from build123d import *

# Parameters (mm, degrees)
SKETCH1_R           = 1.75
BOSS_EXTRUDE1_DEPTH = 5


with BuildPart() as part:
    # Sketch1 → Boss-Extrude1 (new body)
    with BuildSketch(Plane.XY):
        with BuildLine():
            Line((-93.75, -249.14706128), (-98.75, -249.14706128))
            Line((-98.75, -249.14706128), (-98.75, -275.963602955))
            Line((-98.75, -275.963602955), (-93.75, -275.963602955))
            add(Edge.make_bspline(
                [(-93.75, -275.963602955), (-85.328784133, -309.023467032), (-87.242655609, -343.164760507), (-85.696102167, -376.929671114)],
                knots=[0, 0, 0, 0, 1, 1, 1, 1], degree=3))
            Line((-85.696102167, -376.929671114), (82.9, -376.929671114))
            add(Edge.make_bspline(
                [(82.9, -274.035506052), (82.9, -308.333561073), (82.9, -342.631616093), (82.9, -376.929671114)],
                knots=[0, 0, 0, 0, 1, 1, 1, 1], degree=3))
            Line((82.9, -274.035506052), (82.9, -262.713680137))
            ThreePointArc((82.9, -262.713680137), (82.607106781, -262.006573355), (81.9, -261.713680137))
            Line((81.9, -261.713680137), (77.9, -261.713680137))
            add(Edge.make_bspline(
                [(77.9, -261.713680137), (75.588198468, -253.598889885), (76.340151595, -245.239667724), (76.055808767, -236.957982208)],
                knots=[0, 0, 0, 0, 1, 1, 1, 1], degree=3))
            Line((76.055808767, -236.957982208), (-91.666234566, -236.957982208))
            add(Edge.make_bspline(
                [(-93.75, -249.14706128), (-91.542697993, -245.516719889), (-91.581655695, -241.056968833), (-91.666234566, -236.957982208)],
                knots=[0, 0, 0, 0, 1, 1, 1, 1], degree=3))
        make_face()
        with Locations((-96.249351551, -269.713963286)):
            Circle(SKETCH1_R, mode=Mode.SUBTRACT)
        with Locations((-96.243654126, -254.713964368)):
            Circle(SKETCH1_R, mode=Mode.SUBTRACT)
        with Locations((80.4, -267.874593094)):
            Circle(SKETCH1_R, mode=Mode.SUBTRACT)
    extrude(amount=BOSS_EXTRUDE1_DEPTH)


solid = part.part
Geometry: final body of the model. Coordinates: model frame, mm. A direction names the side the tool comes from. Coordinates: 2 decimals unless noted, no trailing zeros. One line per item, written item: value. Start each with the question number.
1) Pin query (flat end, axial travel): P1, Ø2, axis at x = -96.24, y = -254.71, coming from the +Z side; P2, Ø2, axis at y = -310.5, z = 1, coming from the -X side; P3, Ø1.5, axis at y = -362.5, z = 4.5, coming from the -X side; P4, Ø1.5, axis at x = -97.5, z = 1.5, coming from the -Y side. Return the tip coordinate at first contact, or that it passes through.
2) Material intervals for L1, parallel to Y at x = 80.4, z = 1.3; L2, parallel to X at y = -303, z = 3.6; L3, parallel to X at y = -249, z = 1.4, sorted ascending. Write a range as from..to.
3) Reachability of faces 1 (the flat face through (-96, -275.964, 2)), 2 (the flat face through (80, -261.714, 2)), 3 (the flat face through (-9, -306, 0)) from +Z, -Z, +X, -X, +Y, -Y: full face, straight path, thin tool, end or side. Return the list, or none.
4) Cut plane A-A (z = 3.6). Count the separate pieces of the cut face and the enclosed holes in it, then the cut area to 3 significant figures.
5) Draft query along Y for faces 4 (the cylindrical face through (79.01, -268.94, 2.46)), 5 (the flat face through (-98.75, -262, 2)), 6 (the flat face through (-96, -249.147, 2)). Return one class per face: released by +Y, released by -Y, zero draft, split by the parting line, or undercut.
Evaluation:
1. P1: through
1. P2: x = -88.25
1. P3: x = -86.2
1. P4: y = -275.96
2. L1: -376.93..-269.62, -266.12..-261.71
2. L2: -88.91..82.9
2. L3: -93.66..76.21
3. face 1: +Z, -Z, -X, -Y
3. face 2: +Z, -Z, +X, +Y
3. face 3: -Z, +X, -X, +Y, -Y
4. separate pieces: 1
4. enclosed holes: 3
4. area: 24,100 mm^2
5. face 4: undercut
5. face 5: zero draft
5. face 6: released by +Y
